Read the model definition and answer for the solid it produces. Units are mm, in the model's axes. Coordinates: 2 decimals unless noted, no trailing zeros. Order: outer loops, then holes, each group sorted by start corner. A loop starts at its lowest first (then second) coordinate and runs counter-clockwise, first axis right, second up.
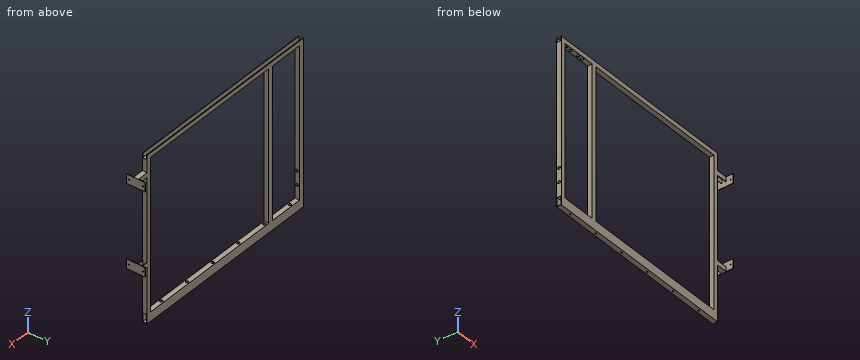
```python
from build123d import *

# Parameters (mm, degrees)
F0_W      = 42
F0_H      = 42
F1_DEPTH  = 1635
F2_W      = 42
F2_H      = 92
F3_DEPTH  = 2125
F7_DEPTH  = 2125
F8_R      = 15
F9_DEPTH  = 50
F10_R     = 15
F11_DEPTH = 250
F13_DEPTH = 116
F14_W     = 200
F14_H     = 100
F14_R     = 6
F15_DEPTH = 4
F16_W     = 50
F16_H     = 50
F16_W_2   = 42
F16_H_2   = 42
F17_DEPTH = 1635
F18_R     = 7
F19_DEPTH = 125
F20_R     = 15
F20_R_2   = 7
F21_DEPTH = 5


# Not quite as in the source:
# - a feature names something its author has since deleted; it is built from what else it names


with BuildPart() as f1:
    # F0 (on Top) → F1 (new body)
    with BuildSketch(Plane.XY):
        Polygon((0, 4), (0, 0), (50, 0), (50, 50), (0, 50), (0, 46), align=None)
        with Locations((25, 25)):
            Rectangle(F0_W, F0_H, mode=Mode.SUBTRACT)
    extrude(amount=F1_DEPTH)


with BuildPart() as f3:
    # F2 (on face) → F3 (new body)
    with BuildSketch(Plane(origin=(0, 0, 0), x_dir=(0, -1, 0), z_dir=(-1, 0, 0))):
        Polygon((0, 0), (-50, 0), (-50, -4), (-50, -96), (-50, -100), (0, -100), align=None)
        with Locations((-25, -50)):
            Rectangle(F2_W, F2_H, mode=Mode.SUBTRACT)
    extrude(amount=-F3_DEPTH)

    # F5: F1 across plane
    add(f1.part.mirror(Plane.YZ.offset(1062.5)))


with BuildPart() as f1_1:
    add(f1.part)

    add(f3.part)  # F7 merges F3
    # F6 (on face) → F7 (join, through all)
    with BuildSketch(Plane(origin=(0, 0, 0), x_dir=(0, -1, 0), z_dir=(-1, 0, 0))):
        Polygon((-46, 1685), (-50, 1685), (-50, 1635), (0, 1635), (0, 1685), (-4, 1685), (-4, 1639), (-46, 1639), align=None)
    extrude(amount=-F7_DEPTH)

    # F8 (on face) → F9 (cut)
    with BuildSketch(Plane.XY.offset(1639)):
        with Locations((315, 25)):
            Circle(F8_R)
        with Locations((155, 25)):
            Circle(F8_R)
        with Locations((255, 25)):
            Circle(F8_R)
        with Locations((95, 25)):
            Circle(F8_R)
    extrude(amount=-F9_DEPTH, mode=Mode.SUBTRACT)

    # F10 (on face) → F11 (cut)
    with BuildSketch(Plane.YZ.offset(50)):
        with Locations((25, 300)):
            Circle(F10_R)
        with Locations((25, 150)):
            Circle(F10_R)
    extrude(amount=-F11_DEPTH, mode=Mode.SUBTRACT)

    # F12 (on face) → F13 (join)
    with BuildSketch(Plane.YZ.offset(2125)):
        Polygon((4, 550), (0, 550), (0, 500), (50, 500), (50, 550), (46, 550), (46, 504), (4, 504), align=None)
        Polygon((0, 1500), (0, 1450), (4, 1450), (4, 1496), (46, 1496), (46, 1450), (50, 1450), (50, 1500), align=None)
    extrude(amount=F13_DEPTH)

    # F14 (on face) → F15 (join)
    with BuildSketch(Plane.YZ.offset(2241)):
        with Locations((25, 1450)):
            Rectangle(F14_W, F14_H)
        with Locations((-50, 1450)):
            Circle(F14_R, mode=Mode.SUBTRACT)
        with Locations((100, 1450)):
            Circle(F14_R, mode=Mode.SUBTRACT)
        with Locations((25, 550)):
            Rectangle(F14_W, F14_H)
        with Locations((-50, 550)):
            Circle(F14_R, mode=Mode.SUBTRACT)
        with Locations((100, 550)):
            Circle(F14_R, mode=Mode.SUBTRACT)
    extrude(amount=F15_DEPTH)

    # F16 (on face) → F17 (join, through all)
    with BuildSketch(Plane.XY):
        with Locations((445, 25)):
            Rectangle(F16_W, F16_H)
        with Locations((445, 25)):
            Rectangle(F16_W_2, F16_H_2, mode=Mode.SUBTRACT)
    extrude(amount=F17_DEPTH)

    # F18 (on face) → F19 (cut)
    with BuildSketch(Plane(origin=(0, 0, -100), x_dir=(1, 0, 0), z_dir=(0, 0, -1))):
        with Locations((150, -25)):
            Circle(F18_R)
        with Locations((500, -25)):
            Circle(F18_R)
        with Locations((850, -25)):
            Circle(F18_R)
        with Locations((1200, -25)):
            Circle(F18_R)
        with Locations((1550, -25)):
            Circle(F18_R)
        with Locations((1900, -25)):
            Circle(F18_R)
    extrude(amount=-F19_DEPTH, mode=Mode.SUBTRACT)

    # F20 (on face) → F21 (cut)
    with BuildSketch(Plane.XY):
        with Locations((500, 25)):
            Circle(F20_R)
        with Locations((500, 25)):
            Circle(F20_R_2, mode=Mode.SUBTRACT)
        with Locations((850, 25)):
            Circle(F20_R)
        with Locations((850, 25)):
            Circle(F20_R_2, mode=Mode.SUBTRACT)
        with Locations((1200, 25)):
            Circle(F20_R)
        with Locations((1200, 25)):
            Circle(F20_R_2, mode=Mode.SUBTRACT)
        with Locations((1550, 25)):
            Circle(F20_R)
        with Locations((1550, 25)):
            Circle(F20_R_2, mode=Mode.SUBTRACT)
        with Locations((1900, 25)):
            Circle(F20_R)
        with Locations((1900, 25)):
            Circle(F20_R_2, mode=Mode.SUBTRACT)
        with Locations((150, 25)):
            Circle(F20_R)
    extrude(amount=-F21_DEPTH, mode=Mode.SUBTRACT)


solid = f1_1.part
```
1) A cutting plane is placed at B-B, the plane x = 776. Determine the outline of the cut face in (y, z), and give its area (3 significant figures).
A:
outline: (0, -100) - (50, -100) - (50, 0) - (0, 0) - close; (0, 1635) - (50, 1635) - (50, 1685) - (46, 1685) - (46, 1639) - (4, 1639) - (4, 1685) - (0, 1685) - close; hole (4, -96) - (46, -96) - (46, -4) - (4, -4) - close
area: 1,700 mm2
2) A cutting plane is placed at A-A, the plane z = 193.5. Determine the outline of the cut face in (x, y).
A:
outline: (0, 0) - (50, 0) - (50, 50) - (0, 50) - close; (420, 0) - (470, 0) - (470, 50) - (420, 50) - close; (2075, 0) - (2125, 0) - (2125, 50) - (2075, 50) - close; hole (4, 4) - (46, 4) - (46, 46) - (4, 46) - close; hole (424, 4) - (466, 4) - (466, 46) - (424, 46) - close; hole (2079, 4) - (2121, 4) - (2121, 46) - (2079, 46) - close
3) Flat-ended cylindrical pins translate along their axes: pin 1 Ø9.5 at (y, z) = (-50, 1450) entering from -X; pin 2 Ø21 at (x, z) = (16, 974) entering from +Y; pin 3 Ø21 at (x, z) = (2102, 1114) entering from -Y. Find the tip coordinate at first contact, or state that the pin passes through.
A:
pin 1: passes through
pin 2: stops at y = 50
pin 3: stops at y = 0
4) Straight lines are drawn through the part: line 1 (X direction, y = 19, z = 417.5); line 2 (Y direction, x = 2243, z = 1450); line 3 (Z direction, x = 1137.5, y = 18). For each, find the intervals that lie inside material, in ascending order.
A:
line 1: x = 0 to 4, 46 to 50, 420 to 424, 466 to 470, 2075 to 2079, 2121 to 2125
line 2: y = -75 to -56, -44 to 94, 106 to 125
line 3: z = -100 to -96, -4 to 0, 1635 to 1639
